Geometry: see drawing. Coordinates: mm, zero at the bounding-box minimum. A direction names the side the tool comes from. Round coordinates to 2 decimals unless told otherwise and drop trailing zeros. Loops run counter-clockwise (first coordinate to the right, second up) from the corner with the lowest first, then second, coordinate; pieces in that order, holes last. Notation, with made-up numbers: M 12,83.5 L 35,83.5 A16 cw 35,111.5 Z; hole C 44,63.25 d9. An arc over 180 degrees is marked long. Answer as a JSON object with one key per item and string values.
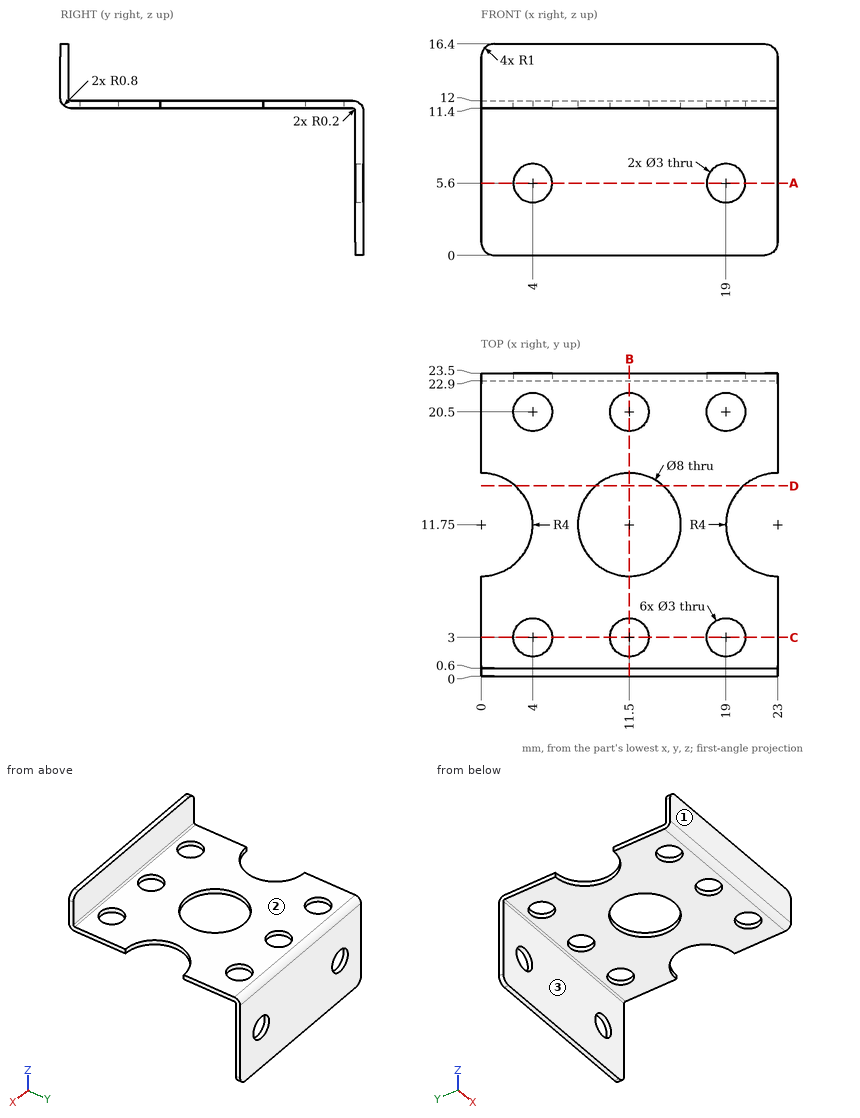
1) Pin query (flat end, axial travel): P1, Ø5.5, axis at x = 6, z = 5, coming from the -Y side; P2, Ø4, axis at y = 19.5, z = 14.5, coming from the -X side (3 decimals); P3, Ø4, axis at x = 11.5, y = 20.5, coming from the -Z side; P4, Ø1, axis at x = 3, z = 13.5, coming from the +Y side. Return the tip coordinate at first contact, or that it passes through.
Results:
{"P1": "y = 22.9", "P2": "through", "P3": "z = 11.4", "P4": "y = 0.6"}
2) Reachability of the marked faces 1, 2 and 3 from +Z, -Z, +X, -X, +Y, -Y: full face, straight path, thin tool, end or side. Return the list, or none.
Results:
{"face 1": "+Z, -Z, +X, -X, -Y", "face 2": "+Z, +X, -X, +Y", "face 3": "-Z, +X, -X, -Y"}
3) Section query D-D (y = 14.75). Return the cut outline in (x, z), and give its area (3 significant figures).
Results:
{"outline": "M 2.65,11.4 L 8.85,11.4 L 8.85,12 L 2.65,12 Z; M 14.15,11.4 L 20.35,11.4 L 20.35,12 L 14.15,12 Z", "area": "7.45 mm2"}
4) Ray query, line 1 (X direction, y = 21, z = 11.75); line 2 (Y direction, x = 11.5, z = 11.65); line 3 (Y direction, x = 12.75, z = 15). Return the intervals inside material, ascending.
Results:
{"line 1": "0 to 2.59, 5.41 to 10.09, 12.91 to 17.59, 20.41 to 23", "line 2": "0.22 to 1.5, 4.5 to 7.75, 15.75 to 19, 22 to 23.36", "line 3": "0 to 0.6"}
5) Section query C-C (y = 3). Return the cut outline in (x, z).
Results:
{"outline": "M 0,11.4 L 2.5,11.4 L 2.5,12 L 0,12 Z; M 5.5,11.4 L 10,11.4 L 10,12 L 5.5,12 Z; M 13,11.4 L 17.5,11.4 L 17.5,12 L 13,12 Z; M 20.5,11.4 L 23,11.4 L 23,12 L 20.5,12 Z"}
6) Section query A-A (z = 5.6). Return the cut outline in (x, y), and give its area (3 significant figures).
Results:
{"outline": "M 0,22.9 L 2.5,22.9 L 2.5,23.5 L 0,23.5 Z; M 5.5,22.9 L 17.5,22.9 L 17.5,23.5 L 5.5,23.5 Z; M 20.5,22.9 L 23,22.9 L 23,23.5 L 20.5,23.5 Z", "area": "10.2 mm2"}
7) Section query B-B (x = 11.5). Return the cut outline in (y, z).
Results:
{"outline": "M 0,12.2 A0.8 ccw 0.8,11.4 L 1.5,11.4 L 1.5,12 L 0.8,12 A0.2 cw 0.6,12.2 L 0.6,16.4 L 0,16.4 Z; M 4.5,11.4 L 7.75,11.4 L 7.75,12 L 4.5,12 Z; M 15.75,11.4 L 19,11.4 L 19,12 L 15.75,12 Z; M 22,11.4 L 22.7,11.4 A0.2 cw 22.9,11.2 L 22.9,0 L 23.5,0 L 23.5,11.2 A0.8 ccw 22.7,12 L 22,12 Z"}
